Print and shaded views of the part. All mm, measured from the part's lowest x, y and z. Round coordinates to 2 decimals unless told otherwise and drop trailing zeros. Write each loop counter-clockwise with the first axis right and the second up, starting at its lowest first coordinate (ties: lowest second). Pieces come first, ordered by that corner, then holes. Notation, with made-up numbers: (62.5, 62.5) - (102.5, 62.5) arc R14 cw to (102.5, 75.5) - close; hole circle Ø9 at (23.5, 7). An arc over 180 degrees is marked (long way). One line per item, written item: value.
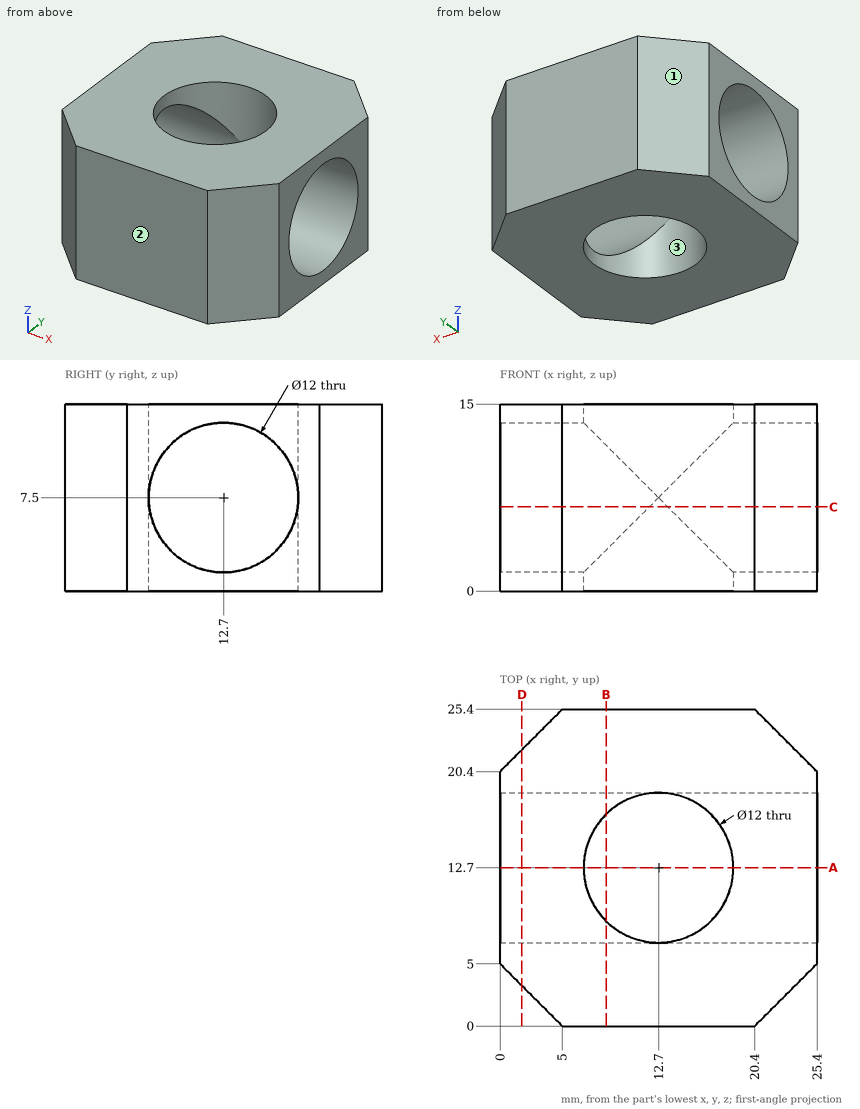
1. Band-saw the part on D-D on x = 1.75. Write the cut outline in (y, z), plus the area to 3 significant figures.
Report:
outline: (3.25, 0) - (22.15, 0) - (22.15, 15) - (3.25, 15) - close; hole circle Ø12 at (12.7, 7.5)
area: 170 mm²
2. Band-saw the part on C-C on z = 6.75. Write the cut outline in (x, y), plus the area to 3 significant figures.
Report:
outline: (0, 5) - (5, 0) - (20.4, 0) - (25.4, 5) - (25.4, 6.75) - (13.45, 6.75) arc R6 cw to (11.95, 6.75) - (0, 6.75) - close; (0, 18.65) - (11.95, 18.65) arc R6 cw to (13.45, 18.65) - (25.4, 18.65) - (25.4, 20.4) - (20.4, 25.4) - (5, 25.4) - (0, 20.4) - close
area: 293 mm²
3. Wall check: probe 1 along Y at (x, z) = (12.7, 2.25); probe 2 along Z at (x, y) = (19.75, 12.7); probe 3 along Y at (x, z) = (5.75, 10.25). Give the ranges that are in metal, low to high. Write a range as [from, to].
Report:
probe 1: [0, 6.7], [18.7, 25.4]
probe 2: [0, 1.5], [13.5, 15]
probe 3: [0, 7.37], [18.03, 25.4]
4. Mould opens along X. For the marked faces 1, 2 and 3 say: released by +X, released by -X, zero draft, split by the parting line, or undercut.
Report:
face 1: released by -X
face 2: zero draft
face 3: undercut
5. Drop a flat-ended pin along its axis: pin 1 (4 mm diameter, centred on x = 17, y = 14.5, fed in from -Z). Give the stop position or say it passes through.
Report:
pin 1: z = 0
6. Band-saw the part on B-B on x = 8.5. Write the cut outline in (y, z).
Report:
outline: (0, 0) - (8.42, 0) - (8.42, 3.3) arc R6 cw to (8.42, 11.7) - (8.42, 15) - (0, 15) - close; (16.98, 0) - (25.4, 0) - (25.4, 15) - (16.98, 15) - (16.98, 11.7) arc R6 cw to (16.98, 3.3) - close
7. Band-saw the part on A-A on y = 12.7. Write the cut outline in (x, z), plus the area to 3 significant figures.
Report:
outline: (0, 0) - (6.7, 0) - (6.7, 1.5) - (0, 1.5) - close; (0, 13.5) - (6.7, 13.5) - (6.7, 15) - (0, 15) - close; (18.7, 0) - (25.4, 0) - (25.4, 1.5) - (18.7, 1.5) - close; (18.7, 13.5) - (25.4, 13.5) - (25.4, 15) - (18.7, 15) - close
area: 40.2 mm²
